from build123d import *

# Parameters (mm, degrees)
SKETCH1_R                               = 49
DISC_PLATE_DEPTH                        = 6
SKETCH2_W                               = 68
SKETCH2_H                               = 14
BOSS_DEPTH                              = 10
SKETCH3_W                               = 62.3
SKETCH3_H                               = 3.2
SPINE_SLOT_DEPTH                        = 10
SKETCH4_W                               = 3
SKETCH4_H                               = 5.5
FILLET1_R                               = 0.2
CBORE_FOR_M5_HEX_HEAD_BOLT1_D           = 3.4
CBORE_FOR_M5_HEX_HEAD_BOLT1_DEPTH       = 5.4
CBORE_FOR_M5_HEX_HEAD_BOLT1_CBORE_D     = 6.2
CBORE_FOR_M5_HEX_HEAD_BOLT1_CBORE_DEPTH = 3.2
CBORE_FOR_M5_HEX_HEAD_BOLT1_TIP         = 1.021463052
SKETCH9_R                               = 2.1
INSERT_HOLES_DEPTH                      = 6.5
SKETCH10_R                              = 7
CABLE_HOLES_DEPTH                       = 72.119617547
CHAMFER1_SIZE                           = 0.5


with BuildPart() as part:
    # Sketch1 → Disc_Plate (new body)
    with BuildSketch(Plane.XY):
        Circle(SKETCH1_R)
    extrude(amount=DISC_PLATE_DEPTH)

    # Sketch2 → Boss (add)
    with BuildSketch(Plane.XY.offset(6)):
        Rectangle(SKETCH2_W, SKETCH2_H)
    extrude(amount=BOSS_DEPTH)

    # Sketch3 → Spine Slot (cut)
    with BuildSketch(Plane.XY.offset(16)):
        Rectangle(SKETCH3_W, SKETCH3_H)
    extrude(amount=-SPINE_SLOT_DEPTH, mode=Mode.SUBTRACT)

    # Sketch4 → Friction_Groove (revolve, cut)
    with BuildSketch(Plane(origin=(0, 0, 0), x_dir=(0, 0, -1), z_dir=(1, 0, 0)), mode=Mode.PRIVATE) as friction_groove_sk:
        with Locations((-3, 49.25)):
            Rectangle(SKETCH4_W, SKETCH4_H)
    revolve(friction_groove_sk.sketch.rotate(Axis((0, 0, 6), (0, 0, -1)), 90), axis=Axis((0, 0, 6), (0, 0, -1)), mode=Mode.SUBTRACT)

    # Fillet1
    fillet1_edges = [part.edges().sort_by_distance(p)[0] for p in [
        (-46.5, 0, 1.5),
        (-46.5, 0, 4.5),
    ]]
    fillet(fillet1_edges, radius=FILLET1_R)

    # CBORE for M5 Hex Head Bolt1
    with Locations(Plane(origin=(0, 7, 0), x_dir=(1, 0, 0), z_dir=(0, 1, 0))):
        with Locations((-25, -11), (25, -11), (11.381423857, 19.171145686)):
            CounterBoreHole(CBORE_FOR_M5_HEX_HEAD_BOLT1_D / 2, CBORE_FOR_M5_HEX_HEAD_BOLT1_CBORE_D / 2, CBORE_FOR_M5_HEX_HEAD_BOLT1_CBORE_DEPTH, depth=CBORE_FOR_M5_HEX_HEAD_BOLT1_DEPTH)
            with Locations((0, 0, -(CBORE_FOR_M5_HEX_HEAD_BOLT1_DEPTH + CBORE_FOR_M5_HEX_HEAD_BOLT1_TIP / 2))):  # 118° drill point
                Cone(0, CBORE_FOR_M5_HEX_HEAD_BOLT1_D / 2, CBORE_FOR_M5_HEX_HEAD_BOLT1_TIP, mode=Mode.SUBTRACT)

    # Sketch9 → Insert_Holes (cut)
    with BuildSketch(Plane(origin=(0, -1.6, 0), x_dir=(1, 0, 0), z_dir=(0, 1, 0))):
        with Locations(Location((-25, -11, 0), (0, 0, 270))):
            Circle(SKETCH9_R)
        with Locations(Location((25, -11, 0), (0, 0, 270))):
            Circle(SKETCH9_R)
    extrude(amount=-INSERT_HOLES_DEPTH, mode=Mode.SUBTRACT)

    # Sketch10 → Cable_Holes (cut, through all)
    with BuildSketch(Plane.XY):
        with Locations((20, 32)):
            Circle(SKETCH10_R)
        with Locations(Location((20, -32, 0), (0, 0, 180))):
            Circle(SKETCH10_R)
        with Locations((-20, -32)):
            Circle(SKETCH10_R)
        with Locations(Location((-20, 32, 0), (0, 0, 180))):
            Circle(SKETCH10_R)
    extrude(amount=CABLE_HOLES_DEPTH, mode=Mode.SUBTRACT)

    # Chamfer1
    chamfer1_edges = [part.edges().sort_by_distance(p)[0] for p in [
        (-49, 0, 0),
        (-49, 0, 6),
        (-13, 32, 6),
        (-13, 32, 0),
        (-27, -32, 6),
        (-27, -32, 0),
        (27, -32, 6),
        (27, -32, 0),
        (13, 32, 6),
        (13, 32, 0),
    ]]
    chamfer(chamfer1_edges, length=CHAMFER1_SIZE)


solid = part.part
Build history of the part. All positions in model axes, mm. A direction names the side the tool comes from. Round coordinates to 2 decimals unless told otherwise and drop trailing zeros. Write each loop counter-clockwise with the first axis right and the second up, starting at its lowest first coordinate (ties: lowest second). Pieces come first, ordered by that corner, then holes. Notation, with made-up numbers: M -16,-32 L -11,-32 A6 cw -11,-25 Z; hole C 33,-14.75 d11. An arc over 180 degrees is marked long. Answer as a JSON object with one key per item and string values. Group by question number.
(1) Flat gauge pins, fed straight in: pin 1 (3.5 mm diameter, centred on y = 0.5, z = 11.5, fed in from +X); pin 2 (16 mm diameter, centred on x = 20, y = 32, fed in from +Z); pin 3 (1.9 mm diameter, centred on x = -26.5, z = 11.5, fed in from +Y); pin 4 (2.5 mm diameter, centred on x = 25, z = 11, fed in from +Y). Where does each tip first touch, or does it go through?
(2) Cut at A-A (x = 0). Give the cut face in (y, z), and give its area (3 significant figures).
(3) Cut at B-B (y = 0). Give the cut face in (x, z).
(4) Cut at C-C (x = -25). Give the number of separate pieces and of enclosed holes in the cut face, and give its area (3 significant figures).
(5) Mould opens along Z. For faces 6 (the flat face through (34, 0, 11)), 7 (the flat face through (-1, 1, 0)), 8 (the cylindrical face through (26.419, -4.262, 9.452)) say: pulls with the +Z half, pulls with the -Z half, needs draft (parallel to the pull), parting line crosses it, or undercut.
(6) Which spindle directions (+Z, -Z, +X, -X, +Y, -Y) get a long thin tool onto all of the face, cutting with end or side? Do faces 1 (the flat face through (0, -7, 11)), 2 (the cylindrical face through (44.35, -13.97, 2.98)), 3 (the flat face through (0, 7, 11)), 4 (the flat face through (26.33, 3.8, 12.33)), 5 (the cylindrical face through (23.43, 2.68, 11.65)). Say none if no direction does.
(7) Drill centre lines: L1, parallel to X at y = 6.3, z = 11; L2, parallel to X at y = 3.3, z = 11; L3, parallel to Y at x = -11.5, z = 12. Where is each one in solid material? Low to high.
Responses:
{
 "1": {"pin 1": "stops at x = 34", "pin 2": "stops at z = 6", "pin 3": "stops at y = 3.8", "pin 4": "passes through"},
 "2": {"outline": "M -49,0.5 L -48.5,0 L 48.5,0 L 49,0.5 L 49,1.5 L 46.7,1.5 A0.2 cw 46.5,1.7 L 46.5,4.3 A0.2 cw 46.7,4.5 L 49,4.5 L 49,5.5 L 48.5,6 L 7,6 L 7,16 L 1.6,16 L 1.6,6 L -1.6,6 L -1.6,16 L -7,16 L -7,6 L -48.5,6 L -49,5.5 L -49,4.5 L -46.7,4.5 A0.2 cw -46.5,4.3 L -46.5,1.7 A0.2 cw -46.7,1.5 L -49,1.5 Z", "area": "681 mm2"},
 "3": {"outline": "M -49,0.5 L -48.5,0 L 48.5,0 L 49,0.5 L 49,1.5 L 46.7,1.5 A0.2 cw 46.5,1.7 L 46.5,4.3 A0.2 cw 46.7,4.5 L 49,4.5 L 49,5.5 L 48.5,6 L 34,6 L 34,16 L 31.15,16 L 31.15,6 L -31.15,6 L -31.15,16 L -34,16 L -34,6 L -48.5,6 L -49,5.5 L -49,4.5 L -46.7,4.5 A0.2 cw -46.5,4.3 L -46.5,1.7 A0.2 cw -46.7,1.5 L -49,1.5 Z"},
 "4": {"separate pieces": "5", "enclosed holes": "0", "area": "427 mm2"},
 "5": {"face 6": "needs draft", "face 7": "pulls with the -Z half", "face 8": "undercut"},
 "6": {"face 1": "+Z, +X, -X, -Y", "face 2": "none", "face 3": "+Z, +X, -X, +Y", "face 4": "+Y", "face 5": "+Y, -Y"},
 "7": {"L1": "x = -34 to -28.1, -21.9 to 21.9, 28.1 to 34", "L2": "x = -34 to -26.7, -23.3 to 23.3, 26.7 to 34", "L3": "y = -7 to -1.6, 1.6 to 7"}
}
